Geometry: see drawing. Coordinates: mm, zero at the bounding-box minimum. A direction names the side the tool comes from. Round coordinates to 2 decimals unless told otherwise and drop trailing zeros. Loops run counter-clockwise (first coordinate to the right, second up) from the corner with the lowest first, then second, coordinate; pieces in that order, holes last. Notation, with made-up numbers: (32, 81.25) - (91, 81.25) arc R24 ccw to (91, 115.25) - close; hole circle Ø11 at (57.5, 40.25). An arc over 180 degrees is marked (long way). Answer in a Markdown table with one row per item. Add a question column.
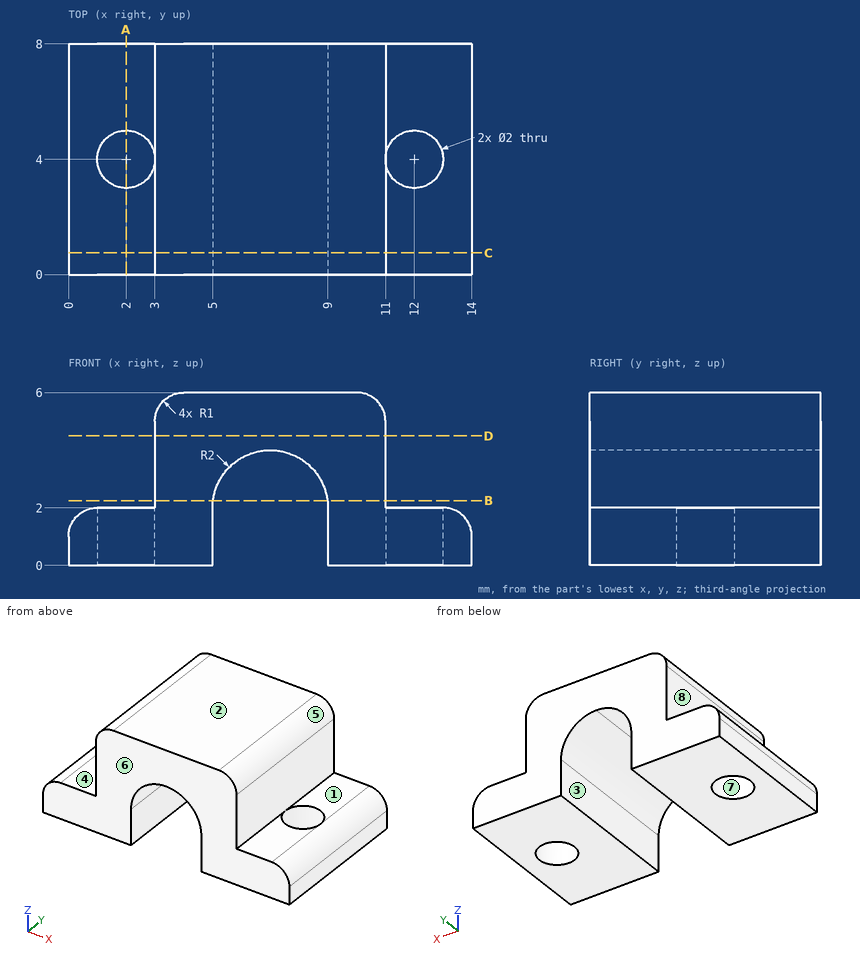
1) Reachability of the marked faces 1, 2, 3 and 4 from +Z, -Z, +X, -X, +Y, -Y: full face, straight path, thin tool, end or side. Return the list, or none.
2) Section A-A, the plane x = 2. Return the cut outline in (y, z), and give its area (3 significant figures).
3) Pull-direction query (X, two-part tool) for the marked faces 5, 6, 7 and 8; classes: pulls with the +X half, pulls with the -X half, needs draft (parallel to the pull), parting line crosses it, or undercut.
4) Material intervals for line 1 along X through (y, z) = (4, 0.8); line 2 along Y through (x, z) = (2, 0.5); line 3 along Z through (x, y) = (2.25, 6.5), sorted ascending. Write a range as from..to.
5) Section B-B, the plane z = 2.25. Return the cut outline in (x, y), and give its area (3 significant figures).
6) Contact query for flat-ended pins moving along their axis: pin 1 Ø1.5 at (y, z) = (2.5, 3.5) entering from +X; pin 2 Ø1.8 at (x, y) = (12, 4) entering from +Z; pin 3 Ø3.5 at (y, z) = (4.5, 3) entering from -X; pin 4 Ø2 at (x, y) = (12.5, 2.5) entering from +Z. Output: stop coordinate, or through.
7) Section D-D, the plane z = 4.5. Return the cut outline in (x, y).
8) Section C-C, the plane y = 0.75. Return the cut outline in (x, z), and give its area (3 significant figures).
Evaluation:
| question | item | result |
|---|---|---|
| 1 | face 1 | +Z, +X, +Y, -Y |
| 1 | face 2 | +Z, +X, -X, +Y, -Y |
| 1 | face 3 | -Z, +Y, -Y |
| 1 | face 4 | +Z, -X, +Y, -Y |
| 2 | outline | (0, 0) - (3, 0) - (3, 2) - (0, 2) - close; (5, 0) - (8, 0) - (8, 2) - (5, 2) - close |
| 2 | area | 12.0 mm² |
| 3 | face 5 | pulls with the +X half |
| 3 | face 6 | needs draft |
| 3 | face 7 | undercut |
| 3 | face 8 | pulls with the -X half |
| 4 | line 1 | x = 0..1, 3..5, 9..11, 13..14 |
| 4 | line 2 | y = 0..3, 5..8 |
| 4 | line 3 | z = 0..2 |
| 5 | outline | (3, 0) - (5.02, 0) - (5.02, 8) - (3, 8) - close; (8.98, 0) - (11, 0) - (11, 8) - (8.98, 8) - close |
| 5 | area | 32.3 mm² |
| 6 | pin 1 | stops at x = 11 |
| 6 | pin 2 | passes through |
| 6 | pin 3 | stops at x = 0.03 |
| 6 | pin 4 | stops at z = 2 |
| 7 | outline | (3, 0) - (11, 0) - (11, 8) - (3, 8) - close |
| 8 | outline | (0, 0) - (5, 0) - (5, 2) arc R2 cw to (9, 2) - (9, 0) - (14, 0) - (14, 1) arc R1 ccw to (13, 2) - (11, 2) - (11, 5) arc R1 ccw to (10, 6) - (4, 6) arc R1 ccw to (3, 5) - (3, 2) - (1, 2) arc R1 ccw to (0, 1) - close |
| 8 | area | 44.9 mm² |
